CAD build for the part. Positions are in the model's coordinates, mm. A direction names the side the tool comes from. Round coordinates to 2 decimals unless told otherwise and drop trailing zeros. Loops run counter-clockwise (first coordinate to the right, second up) from the corner with the lowest first, then second, coordinate; pieces in that order, holes last.
```python
from build123d import *

# Parameters (mm, degrees)
BOSS_EXTRUDE1_DEPTH = 4.4
SKETCH2_R           = 2.65
CUT_EXTRUDE1_DEPTH  = 4
SKETCH5_W           = 13.2
SKETCH5_H           = 32.1
SKETCH5_R           = 2.65
SKETCH5_R_2         = 3.9
BOSS_EXTRUDE5_DEPTH = 1
SKETCH7_W           = 13.2
SKETCH7_H           = 8
SKETCH7_R           = 1.65
BOSS_EXTRUDE7_DEPTH = 5.4


with BuildPart() as part:
    # Sketch1 → Boss-Extrude1 (new body)
    with BuildSketch(Plane(origin=(0, 0, 0), x_dir=(1, 0, 0), z_dir=(0, 1, 0))):
        with BuildLine():
            ThreePointArc((8.894356871, 11.522321429), (11.17380815, 9.48621778), (12.179473661, 6.6))
            Line((12.179473661, 6.6), (12.2, 6.6))
            Line((12.2, 6.6), (12.2, 22.5))
            Line((12.2, 22.5), (12.2, 27.3))
            Line((12.2, 27.3), (-1, 27.3))
            Line((-1, 27.3), (-1, -4.8))
            Line((-1, -4.8), (12.2, -4.8))
            Line((12.2, -4.8), (12.2, 0))
            Line((12.2, 0), (12.2, 5.6))
            Line((12.2, 5.6), (12.179473661, 5.6))
            ThreePointArc((12.179473661, 5.6), (2.71378222, 1.02619185), (3.305643129, 11.522321429))
            ThreePointArc((3.305643129, 11.522321429), (6.1, 14.5), (8.894356871, 11.522321429))
        make_face()
    extrude(amount=BOSS_EXTRUDE1_DEPTH)

    # Sketch2 → Cut-Extrude1 (cut)
    with BuildSketch(Plane(origin=(0, 4.4, 0), x_dir=(1, 0, 0), z_dir=(0, 1, 0))):
        with Locations((2.470606111, 17.8)):
            Circle(SKETCH2_R)
    extrude(amount=-CUT_EXTRUDE1_DEPTH, mode=Mode.SUBTRACT)

    # Sketch5 → Boss-Extrude5 (add)
    with BuildSketch(Plane(origin=(0, 4.4, 0), x_dir=(1, 0, 0), z_dir=(0, 1, 0))):
        with Locations((5.6, 11.25)):
            Rectangle(SKETCH5_W, SKETCH5_H)
        with Locations((2.470606111, 17.8)):
            Circle(SKETCH5_R, mode=Mode.SUBTRACT)
        with Locations((6.1, 6.1)):
            Circle(SKETCH5_R_2, mode=Mode.SUBTRACT)
    extrude(amount=BOSS_EXTRUDE5_DEPTH)

    # Sketch7 → Boss-Extrude7 (add)
    with BuildSketch(Plane(origin=(0, 5.4, 0), x_dir=(1, 0, 0), z_dir=(0, 1, 0))):
        with Locations((5.6, -8.8)):
            Rectangle(SKETCH7_W, SKETCH7_H)
        with Locations((8.6, -8.8)):
            Circle(SKETCH7_R, mode=Mode.SUBTRACT)
        with Locations((2.6, -8.8)):
            Circle(SKETCH7_R, mode=Mode.SUBTRACT)
        with Locations((5.6, 31.3)):
            Rectangle(SKETCH7_W, SKETCH7_H)
        with Locations((8.6, 31.3)):
            Circle(SKETCH7_R, mode=Mode.SUBTRACT)
        with Locations((2.6, 31.3)):
            Circle(SKETCH7_R, mode=Mode.SUBTRACT)
    extrude(amount=-BOSS_EXTRUDE7_DEPTH)


solid = part.part
```
Item 1: 3-axis set-ups, long thin cutter, end or side, ignore diameter. For faces 1 (the cylindrical face through (11.15, 2.17, -9.52)), 2 (the cylindrical face through (2.2, 2.7, -29.7)), 3 (the flat face through (2, 0.4, -18)): which of +Z, -Z, +X, -X, +Y, -Y reach the whole face in a straight line?
Answers follow:
face 1: -Y
face 2: +Y, -Y
face 3: +Y
Item 2: Cut at C-C, the plane y = 4.9. Give the cut face in (x, z), plus the area to 3 significant figures.
Answers follow:
outline: (-1, -35.3) - (12.2, -35.3) - (12.2, 12.8) - (-1, 12.8) - close; hole circle Ø5.3 at (2.47, -17.8); hole circle Ø3.3 at (2.6, -31.3); hole circle Ø3.3 at (2.6, 8.8); hole circle Ø7.8 at (6.1, -6.1); hole circle Ø3.3 at (8.6, -31.3); hole circle Ø3.3 at (8.6, 8.8)
area: 531 mm2
Item 3: Two-plate mould, pull along X, no slides. Class faces 4 (the flat face through (6, 3, 12.8)), 5 (the flat face through (12.2, 3, -11)), 6 (the flat face through (6, 4.4, -11)): released by +X, released by -X, zero draft, split by the parting line, or undercut.
Answers follow:
face 4: zero draft
face 5: released by +X
face 6: undercut
Item 4: Cut at A-A, the plane z = -31.3. Give the cut face in (x, y), plus the area to 3 significant figures.
Answers follow:
outline: (-1, 0) - (0.95, 0) - (0.95, 5.4) - (-1, 5.4) - close; (4.25, 0) - (6.95, 0) - (6.95, 5.4) - (4.25, 5.4) - close; (10.25, 0) - (12.2, 0) - (12.2, 5.4) - (10.25, 5.4) - close
area: 35.6 mm2
Item 5: Cut at D-D, the plane z = -6.1. Give the cut face in (x, y).
Answers follow:
outline: (-1, 0) - (0, 0) - (0, 4.4) - (2.2, 4.4) - (2.2, 5.4) - (-1, 5.4) - close; (10, 4.4) - (12.2, 4.4) - (12.2, 5.4) - (10, 5.4) - close
Item 6: Flat gauge pins, fed straight in: P1, Ø2.5, axis at x = 2.5, z = -17.5, coming from the +Y side; P2, Ø2.5, axis at x = 8.6, z = -31.3, coming from the -Y side. Where does each tip first touch, or does it go through?
Answers follow:
P1: stops at y = 0.4
P2: passes through
Item 7: Probe line 1 (X direction, y = 2.65, z = 8.8); line 2 (Z direction, x = 9.25, y = 3.1); line 3 (Z direction, x = 7.75, y = 5.25). List the from-to ranges inside material, lowest first.
Answers follow:
line 1: x = -1 to 0.95, 4.25 to 6.95, 10.25 to 12.2
line 2: z = -35.3 to -32.82, -29.78 to -11.32, -0.88 to 7.28, 10.32 to 12.8
line 3: z = -35.3 to -32.71, -29.89 to -9.63, -2.57 to 7.39, 10.21 to 12.8
Item 8: Cut at B-B, the plane x = 6.1. Give the cut face in (y, z).
Answers follow:
outline: (0, -35.3) - (5.4, -35.3) - (5.4, -10) - (4.4, -10) - (4.4, -14.5) - (0, -14.5) - close; (0, 0) - (4.4, 0) - (4.4, -2.2) - (5.4, -2.2) - (5.4, 12.8) - (0, 12.8) - close
